Work out the finished part from the listing and answer in its coordinate system (mm). Give positions to 0.01 mm unless a question says otherwise; leave off trailing zeros. Write each loop counter-clockwise with the first axis right and the second up, starting at its lowest first coordinate (ties: lowest second). Pieces come first, ordered by that corner, then holes.
1) Find section B-B (x = 12.5). Determine the outline of the cut face in (y, z), plus the area to 3 significant figures.
2) Given pin 1 Ø5 at (x, y) = (32.5, 10.5) entering from -Z; pin 2 Ø1.5 at (y, z) = (13.5, -63) entering from +X; pin 3 Ø1 at (x, y) = (-6.5, 10.5) entering from -Z, each flat-ended and moving along its own axis, determine where each tip first touches the part or whether it passes through.
3) Find section A-A (y = 9). Determine the outline of the cut face in (x, z).
4) Straight lines are drawn through the part: probe 1 along Z at (x, y) = (-62, 8.5); probe 2 along X at (y, z) = (4, -65); probe 3 along Z at (x, y) = (-34.5, 4.5). For each, find the intervals that lie inside material, in ascending order.
5) Find section C-C (z = -56). Determine the outline of the cut face in (x, y).
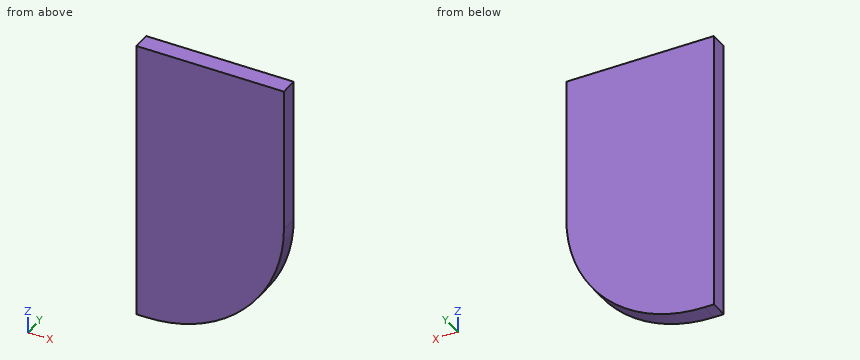
```python
from build123d import *

# Parameters (mm, degrees)
BOSS_EXTRUDE1_DEPTH = 18


with BuildPart() as part:
    # Sketch1 → Boss-Extrude1 (new body)
    with BuildSketch(Plane(origin=(0, 0, 0), x_dir=(1, 0, 0), z_dir=(0, 1, 0))):
        with BuildLine():
            Line((75, -144), (-75, -144))
            Line((-75, -144), (-75, 144))
            Line((-75, 144), (-65, 144))
            ThreePointArc((-65, 144), (33.994949366, 102.994949366), (75, 4))
            Line((75, 4), (75, -144))
        make_face()
    extrude(amount=BOSS_EXTRUDE1_DEPTH)


solid = part.part
```
Results:
1. outline: (0, -120.59) - (18, -120.59) - (18, 144) - (0, 144) - close
1. area: 4,760 mm2
2. pin 1: stops at z = -106.83
2. pin 2: stops at x = 62.31
2. pin 3: stops at z = -131.42
3. outline: (-75, -144) - (-65, -144) arc R140 ccw to (75, -4) - (75, 144) - (-75, 144) - close
4. probe 1: z = -143.97 to 144
4. probe 2: x = -75 to 61.01
4. probe 3: z = -140.64 to 144
5. outline: (-75, 0) - (64.98, 0) - (64.98, 18) - (-75, 18) - close
